```python
from build123d import *

# Parameters (mm, degrees)
F0_W      = 100
F0_H      = 50
F0_W_2    = 90
F0_H_2    = 40
F1_DEPTH  = 7.5
F2_R      = 2.5
F3_DEPTH  = 50.001
F4_W      = 100
F4_H      = 50
F4_W_2    = 90
F4_H_2    = 40
F5_DEPTH  = 10
F7_DEPTH  = 2.5
F8_R      = 1.5
F9_DEPTH  = 1
F10_R     = 1.5
F11_DEPTH = 1
F13_DEPTH = 27.501


with BuildPart() as f1:
    # F0 (on Top) → F1 (new body, symmetric)
    with BuildSketch(Plane.XY):
        Rectangle(F0_W, F0_H)
        Rectangle(F0_W_2, F0_H_2, mode=Mode.SUBTRACT)
    extrude(amount=F1_DEPTH, both=True)

    # F2 (on face) → F3 (cut, through all)
    with BuildSketch(Plane.XZ.offset(25)):
        Circle(F2_R)
        with Locations((-30, 0)):
            Circle(F2_R)
        with Locations((30, 0)):
            Circle(F2_R)
    extrude(amount=-F3_DEPTH, mode=Mode.SUBTRACT)

    # F4 (on face) → F5 (join)
    with BuildSketch(Plane(origin=(0, 0, -7.5), x_dir=(1, 0, 0), z_dir=(0, 0, -1))):
        Rectangle(F4_W, F4_H)
        Rectangle(F4_W_2, F4_H_2, mode=Mode.SUBTRACT)
        Rectangle(F4_W_2, F4_H_2)
    extrude(amount=F5_DEPTH)

    # F6 (on Front) → F7 (join, symmetric)
    with BuildSketch(Plane.XZ):
        with BuildLine():
            Line((-70.0356467673, 16.4644660941), (-50.0356467673, -3.5355339059))
            ThreePointArc((-50.0356467673, -3.5355339059), (-44.5866956996, -4.6193976626), (-41.5001128614, 0))
            Line((-41.5001128614, 0), (-41.5001128614, 20))
            ThreePointArc((-41.5001128614, 20), (-42.9645789555, 23.5355339059), (-46.5001128614, 25))
            Line((-46.5001128614, 25), (-66.5001128614, 25))
            ThreePointArc((-66.5001128614, 25), (-71.119510524, 21.9134171618), (-70.0356467673, 16.4644660941))
        make_face()
    extrude(amount=F7_DEPTH, both=True)

    # F8 (on face) → F9 (cut)
    with BuildSketch(Plane.XZ.offset(2.5)):
        with Locations((-66.5001128614, 20)):
            Circle(F8_R)
    extrude(amount=-F9_DEPTH, mode=Mode.SUBTRACT)

    # F10 (on face) → F11 (cut)
    with BuildSketch(Plane(origin=(0, 2.5, 0), x_dir=(-1, 0, 0), z_dir=(0, 1, 0))):
        with Locations((66.5001128614, 20)):
            Circle(F10_R)
    extrude(amount=-F11_DEPTH, mode=Mode.SUBTRACT)

    # F12 (on face) → F13 (cut, through all)
    with BuildSketch(Plane.XZ.offset(2.5)):
        Polygon((-60.0356467673, 12.4644660941), (-66.0356467673, 12.4644660941), (-60.0356467673, 6.4644660941), align=None)
    extrude(amount=-F13_DEPTH, mode=Mode.SUBTRACT)


solid = f1.part
```
Here's how the part is built. I have some questions about the finished solid (model axes, mm). A direction names the side the tool comes from. Coordinates: 2 decimals unless noted, no trailing zeros. Write each loop counter-clockwise with the first axis right and the second up, starting at its lowest first coordinate (ties: lowest second). Pieces come first, ordered by that corner, then holes. Notation, with made-up numbers: M 75.5,61.25 L 121.5,61.25 A27 cw 121.5,85.25 Z; hole C 73.25,-12 d10. An arc over 180 degrees is marked long. Answer as CSV lines item,"result". Start each with the question number.
Q1. Suppose I cut it at C-C, the plane x = 17.5. List the corners of the cut face in (y, z) for me, then the cut area to 3 significant figures.
Q2. Will these pins go through, and if not, where does the flat tip stop? pin 1 Ø2.5 at (y, z) = (-0.5, 10) entering from -X; pin 2 Ø6 at (y, z) = (-9.5, -2) entering from -X; pin 3 Ø4 at (x, z) = (0, 0) entering from +Y; pin 4 Ø5.5 at (y, z) = (-0.5, 14) entering from +X.
Q3. Suppose I cut it at D-D, the plane z = -15. List the corners of the cut face in (x, y) for me, then the cut area to 3 significant figures.
Q4. For faces 5 (the cylindrical face through (-67.307, 2.007, 21.265)), 6 (the flat face through (-55.106, -0.035, 1.534)), 7 (the flat face through (-1, 20, 3)), which set-ups out of +Z, -Z, +X, -X, +Y, -Y let a thin tool reach every point of the face, with its end or its side?
Q5. I need wall thicknesses on probe 1 along Z at (x, y) = (30, -23.25); probe 2 along Y at (x, z) = (43, -1); probe 3 along X at (y, z) = (-19, 3). Which ranges of each line are inside material? Lowest first, please. Write a range as [from, to].
Q6. Suppose I cut it at B-B, the plane y = 14. List the corners of the cut face in (x, z) for me.
Q7. If we mould it in two halves opening along Z, with no side actions, what happens to faces 1 (the flat face through (-63, 0, 12.464)), 2 (the flat face through (-60.036, 0, 9)), 3 (the cylindrical face through (-32.5, -22.5, 0.1)), 4 (the cylindrical face through (-68, -2, 20))? For each: pulls with the +Z half, pulls with the -Z half, needs draft (parallel to the pull), parting line crosses it, or undercut.
Q8. Suppose I cut it at A-A, the plane x = -30. List the corners of the cut face in (y, z) for me, then the cut area to 3 significant figures.
Entries:
1,outline,"M -25,-17.5 L 25,-17.5 L 25,7.5 L 20,7.5 L 20,-7.5 L -20,-7.5 L -20,7.5 L -25,7.5 Z"
1,area,"650 mm²"
2,pin 1,"stops at x = -60.04"
2,pin 2,"stops at x = -50"
2,pin 3,"passes through"
2,pin 4,"stops at x = -41.5"
3,outline,"M -50,-25 L 50,-25 L 50,25 L -50,25 Z"
3,area,"5,000 mm²"
4,face 5,"+Y"
4,face 6,"-Z, -X, +Y, -Y"
4,face 7,"+Z"
5,probe 1,"z = [-17.5, -2.5], [2.5, 7.5]"
5,probe 2,"y = [-25, -20], [20, 25]"
5,probe 3,"x = [-50, -45], [45, 50]"
6,outline,"M -50,-17.5 L 50,-17.5 L 50,7.5 L 45,7.5 L 45,-7.5 L -45,-7.5 L -45,7.5 L -50,7.5 Z"
7,face 1,"pulls with the -Z half"
7,face 2,"needs draft"
7,face 3,"undercut"
7,face 4,"undercut"
8,outline,"M -25,-17.5 L 25,-17.5 L 25,-2.5 L 20,-2.5 L 20,-7.5 L -20,-7.5 L -20,-2.5 L -25,-2.5 Z; M -25,2.5 L -20,2.5 L -20,7.5 L -25,7.5 Z; M 20,2.5 L 25,2.5 L 25,7.5 L 20,7.5 Z"
8,area,"600 mm²"
